from build123d import *

# Parameters (mm, degrees)
SKETCH1_R           = 4.25
SKETCH1_R_2         = 1.75
BOSS_EXTRUDE1_DEPTH = 5
SKETCH2_W           = 10
SKETCH2_H           = 5
BOSS_EXTRUDE2_DEPTH = 16
BOSS_EXTRUDE4_START = -15
SKETCH2_2_W         = 10
SKETCH2_2_H         = 5
BOSS_EXTRUDE4_DEPTH = 4
BOSS_EXTRUDE5_DEPTH = 10
BOSS_EXTRUDE6_DEPTH = 10
FILLET7_R           = 2
SKETCH8_W           = 24.049628059
SKETCH8_H           = 16.756852772
CUT_EXTRUDE1_DEPTH  = 6
SKETCH9_R           = 1.7
CUT_EXTRUDE2_DEPTH  = 10.15756


with BuildPart() as part:
    # Sketch1 → Boss-Extrude1 (new body)
    with BuildSketch(Plane(origin=(0, 0, 0), x_dir=(1, 0, 0), z_dir=(0, 1, 0))):
        with BuildLine():
            Line((-7.5, -10), (-7.5, 10))
            ThreePointArc((-7.5, 10), (0, 17.5), (7.5, 10))
            Line((7.5, 10), (7.5, -10))
            ThreePointArc((7.5, -10), (0, -17.5), (-7.5, -10))
        make_face()
        Circle(SKETCH1_R, mode=Mode.SUBTRACT)
        with Locations((0, 10)):
            Circle(SKETCH1_R_2, mode=Mode.SUBTRACT)
        with Locations((0, -10)):
            Circle(SKETCH1_R_2, mode=Mode.SUBTRACT)
    extrude(amount=BOSS_EXTRUDE1_DEPTH)

    # Sketch2 → Boss-Extrude2 (add)
    with BuildSketch(Plane(origin=(7.5, 0, 0), x_dir=(0, 0, -1), z_dir=(1, 0, 0))):
        with Locations((-5, 2.5)):
            Rectangle(SKETCH2_W, SKETCH2_H)
    extrude(amount=BOSS_EXTRUDE2_DEPTH)

    # Sketch2_2 → Boss-Extrude4 (add)
    with BuildSketch(Plane(origin=(7.5, 0, 0), x_dir=(0, 0, -1), z_dir=(1, 0, 0)).offset(BOSS_EXTRUDE4_START)):
        with Locations((-5, 2.5)):
            Rectangle(SKETCH2_2_W, SKETCH2_2_H)
    extrude(amount=-BOSS_EXTRUDE4_DEPTH)

    # Sketch4 → Boss-Extrude5 (add)
    with BuildSketch(Plane.XY.offset(10)):
        Polygon((-9.312783412, 30), (-11.5, 5), (-7.5, 5), (-5.312783412, 30), align=None)
        Polygon((15.091825482, 30), (19.5, 5), (23.5, 5), (19.091825482, 30), align=None)
    extrude(amount=-BOSS_EXTRUDE5_DEPTH)

    # Sketch5 → Boss-Extrude6 (add)
    with BuildSketch(Plane.XY.offset(10)):
        with BuildLine():
            Line((19.091825482, 30), (-9.312783412, 30))
            ThreePointArc((-9.312783412, 30), (-13.921057054, 35.078779792), (-9.312783412, 40.157559584))
            Line((-9.312783412, 40.157559584), (19.091825482, 40.157559584))
            Line((19.091825482, 40.157559584), (18.56284454, 37.513443833))
            Line((18.56284454, 37.513443833), (-9.050317421, 37.513443833))
            ThreePointArc((-9.050317421, 37.513443833), (-11.307039338, 35.256721917), (-9.050317421, 33))
            Line((-9.050317421, 33), (18.56284454, 33))
            Line((18.56284454, 33), (19.091825482, 30))
        make_face()
    extrude(amount=-BOSS_EXTRUDE6_DEPTH)

    # Fillet7
    fillet7_edges = [part.edges().sort_by_distance(p)[0] for p in [
        (7.5, 2.5, 0),
        (-7.5, 2.5, 0),
        (-7.5, 2.5, 10),
        (7.5, 2.5, 10),
    ]]
    fillet(fillet7_edges, radius=FILLET7_R)

    # Sketch8 → Cut-Extrude1 (cut, through all)
    with BuildSketch(Plane(origin=(0, 5, 0), x_dir=(1, 0, 0), z_dir=(0, 1, 0))):
        with Locations((0.399485588, 10.378426386)):
            Rectangle(SKETCH8_W, SKETCH8_H)
    extrude(amount=-CUT_EXTRUDE1_DEPTH, mode=Mode.SUBTRACT)

    # Sketch9 → Cut-Extrude2 (cut)
    with BuildSketch(Plane(origin=(0, 40.157559584, 0), x_dir=(1, 0, 0), z_dir=(0, 1, 0))):
        with Locations((-1.312783412, -5)):
            Circle(SKETCH9_R)
        with Locations((8.687216588, -5)):
            Circle(SKETCH9_R)
    extrude(amount=-CUT_EXTRUDE2_DEPTH, mode=Mode.SUBTRACT)


solid = part.part
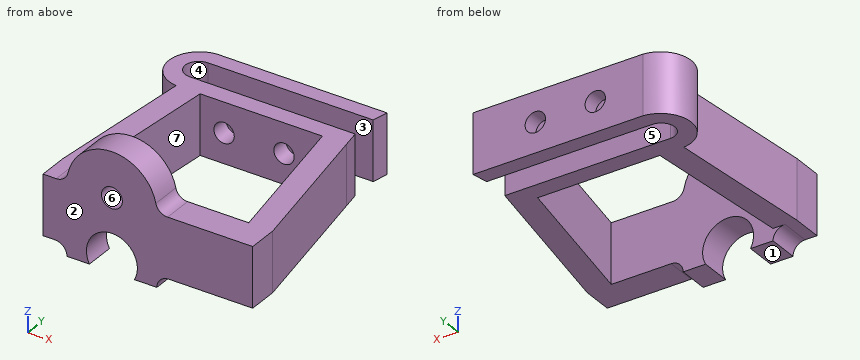
Can you work these out from the model? Positions are in its coordinate system, mm. Face numbers are marked on the shaded views. A direction names the side the tool comes from. Give positions to 0.01 mm unless a question says otherwise; leave off trailing zeros. Write each loop counter-clockwise with the first axis right and the second up, starting at its lowest first coordinate (ties: lowest second). Pieces come first, ordered by that corner, then holes. Notation, with made-up numbers: M 39.25,16 L 94.25,16 A10 cw 94.25,28 Z; hole C 44,-7.5 d4. An arc over 180 degrees is marked long. Answer in a Markdown table with one row per item. Add a question column.
Item 1: On a 3-axis mill with a long thin cutter (end or side, diameter ignored), from which of +Z, -Z, +X, -X, +Y, -Y can I reach the whole of each face in a straight line? I mean the marked faces 5, 6 and 7. Say none if no direction works.
Item 2: Imagine slicing it at D-D, the plane y = 32. Write out the boundary of the cut face in (x, z).
Item 3: We'd pull the mould along Y, two halves only. Please class the marked faces 1, 2, 3 and 4: released by +Y, released by -Y, zero draft, split by the parting line, or undercut.
Item 4: Imagine slicing it at C-C, the plane x = -0.5. Write out the boundary of the cut face in (y, z), plus the area to 3 significant figures.
Item 5: For pin 1 Ø18.5 at (x, y) = (2.5, 18) entering from +Z; pin 2 Ø7.5 at (x, z) = (0, 0) entering from -Y; pin 3 Ø6 at (y, z) = (23.5, 9) entering from -X, each with a flat end and sliding along its axis, tell me the tip position at first contact or that it passes through.
Item 6: Please list where these lines run through material, in increasing order: L1, parallel to Y at x = 4, z = 2.25; L2, parallel to Z at x = 0, y = 2.2; L3, parallel to Y at x = -8, z = 6.75.
Item 7: Imagine slicing it at B-B, the plane x = 18. Write out the boundary of the cut face in (y, z).
Item 8: Imagine slicing it at A-A, the plane z = 5. State how many separate pieces and enclosed holes the cut face has, plus the area to 3 significant figures.
Evaluation:
| question | item | result |
|---|---|---|
| 1 | face 5 | +Z, -Z, +X |
| 1 | face 6 | -Y |
| 1 | face 7 | +Z, -Z |
| 2 | outline | M -12.89,0 L 18.74,0 L 18.74,10 L -12.89,10 Z; hole C -1.31,5 d3.4; hole C 8.69,5 d3.4 |
| 3 | face 1 | zero draft |
| 3 | face 2 | released by -Y |
| 3 | face 3 | undercut |
| 3 | face 4 | undercut |
| 4 | outline | M 0,4.22 L 5,4.22 L 5,8.32 L 0,8.32 Z; M 0,11.68 L 5,11.68 L 5,17.48 L 0,17.48 Z; M 30,0 L 33,0 L 33,3.51 L 30,3.51 Z; M 30,6.49 L 33,6.49 L 33,10 L 30,10 Z; M 37.51,0 L 40.16,0 L 40.16,3.51 L 37.51,3.51 Z; M 37.51,6.49 L 40.16,6.49 L 40.16,10 L 37.51,10 Z |
| 4 | area | 89.1 mm² |
| 5 | pin 1 | stops at z = 10 |
| 5 | pin 2 | stops at y = 30 |
| 5 | pin 3 | stops at x = -10.14 |
| 6 | L1 | y = 0 to 5, 30 to 33, 37.51 to 40.16 |
| 6 | L2 | z = 4.25 to 8.25, 11.75 to 17.5 |
| 6 | L3 | y = 0 to 33, 37.51 to 40.16 |
| 7 | outline | M 0,0 L 5,0 L 5,10 L 0,10 Z; M 13.51,0 L 33,0 L 33,10 L 13.51,10 Z; M 37.51,0 L 40.16,0 L 40.16,10 L 37.51,10 Z |
| 8 | separate pieces | 4 |
| 8 | enclosed holes | 0 |
| 8 | area | 524 mm² |
